The listing builds one solid part. Answer for the finished solid, in the listing's coordinates (mm). A direction names the side the tool comes from. Coordinates: 2 decimals unless noted, no trailing zeros. Order: outer loops, then holes, each group sorted by start corner. A loop starts at its lowest first (then second) coordinate and runs counter-clockwise, first axis right, second up. Notation, with made-up numbers: (32.5, -14.75) -> (44.5, -14.75) arc R24 ccw to (44.5, 0.25) -> close; hole circle Ø9 at (13.25, 54.5). An arc over 180 degrees is marked (long way). One line per question, with ' | ' between items.
from build123d import *

# Parameters (mm, degrees)
BODY_DEPTH          = 160
SKETCH2_R           = 5
PIN_HOLE_DEPTH      = 178.270979012
LPATTERN1_COUNT     = 5
LPATTERN1_PITCH     = 30
SKETCH3_W           = 130
SKETCH3_H           = 170
SKETCH3_W_2         = 100
SKETCH3_H_2         = 150
SPINE_DEPTH         = 40
SKETCH10_W          = 300
SKETCH10_H          = 50
SKETCH10_W_2        = 50
SKETCH10_H_2        = 20
BOSS_EXTRUDE5_DEPTH = 20
CUT_EXTRUDE2_REACH  = 553.549
SKETCH11_W          = 52.942098854
SKETCH11_H          = 11.117065858


with BuildPart() as part:
    # Sketch1 → body (new body)
    with BuildSketch(Plane(origin=(0, 0, 0), x_dir=(1, 0, 0), z_dir=(0, 1, 0))):
        Polygon((65, 20), (-65, 20), (-65, 10), (-55, 10), (-55, -10), (-65, -10), (-65, -20), (65, -20), (65, -10), (55, -10), (55, 10), (65, 10), align=None)
    extrude(amount=BODY_DEPTH)

    # Sketch2 → pin hole (cut, through all)
    with BuildSketch(Plane.XY.offset(20)):
        with Locations((0, 10)):
            Circle(SKETCH2_R)
    pin_hole = extrude(amount=-PIN_HOLE_DEPTH, mode=Mode.SUBTRACT)

    # LPattern1: pin hole ×5
    with Locations(*[(0, i * LPATTERN1_PITCH, 0) for i in range(1, LPATTERN1_COUNT)]):
        add(pin_hole, mode=Mode.SUBTRACT)

    # Sketch3 → spine (add)
    with BuildSketch(Plane.XY.offset(20)):
        with Locations((0, 245)):
            Rectangle(SKETCH3_W, SKETCH3_H)
        with Locations((0, 405)):
            Rectangle(SKETCH3_W_2, SKETCH3_H_2)
    extrude(amount=-SPINE_DEPTH)

    # Sweep4: sweep along a path in Sketch8
    with BuildLine(Plane(origin=(0, 480, 0), x_dir=(1, 0, 0), z_dir=(0, 1, 0))) as sweep4_path:
        ThreePointArc((0, -20), (126.004292483, -12.029696267), (250, 11.754163448))
    # Sketch6<6> → Sweep4 (sweep)
    with BuildSketch(Plane(origin=(0, 0, 0), x_dir=(0, 0, -1), z_dir=(1, 0, 0))):
        Polygon((-70, 480), (-55, 480), (-55, 470), (-35, 470), (-35, 480), (-20, 480), (-20, 430), (-35, 430), (-35, 440), (-55, 440), (-55, 430), (-70, 430), align=None)
    sweep(path=sweep4_path.line)

    # Sketch10 → Boss-Extrude5 (add)
    with BuildSketch(Plane.XY.offset(20)):
        with Locations((0, 455)):
            Rectangle(SKETCH10_W, SKETCH10_H)
        with Locations((-105, 455)):
            Rectangle(SKETCH10_W_2, SKETCH10_H_2, mode=Mode.SUBTRACT)
        with Locations((105, 455)):
            Rectangle(SKETCH10_W_2, SKETCH10_H_2, mode=Mode.SUBTRACT)
    extrude(amount=-BOSS_EXTRUDE5_DEPTH)

    # Sketch11 → Cut-Extrude2 (cut, up to next)
    with BuildSketch(Plane(origin=(0, 480, 0), x_dir=(1, 0, 0), z_dir=(0, 1, 0)), mode=Mode.PRIVATE) as cut_extrude2_sk1:
        with Locations((103.759397545, -17.786929586)):
            Rectangle(SKETCH11_W, SKETCH11_H)
    cut_extrude2_tool1 = extrude(cut_extrude2_sk1.sketch, amount=-CUT_EXTRUDE2_REACH, mode=Mode.PRIVATE) & part.part
    add(cut_extrude2_tool1.solids().sort_by_distance((103.759398, 480, 17.78693))[0], mode=Mode.SUBTRACT)


solid = part.part
Item 1: Section A-A, the plane x = -93 is taken. Give the vertices of the cut face in (y, z), plus the area to 3 significant figures.
Computed values:
outline: (430, 0) -> (445, 0) -> (445, 20) -> (430, 20) -> close; (465, 0) -> (480, 0) -> (480, 20) -> (465, 20) -> close | area: 600 mm^2
Item 2: Section B-B, the plane y = 263 is taken. Give the vertices of the cut face in (x, z).
Computed values:
outline: (-65, -20) -> (65, -20) -> (65, 20) -> (-65, 20) -> close
Item 3: Section C-C, the plane x = 235 is taken. Give the vertices of the cut face in (y, z), plus the area to 3 significant figures.
Computed values:
outline: (430, -8) -> (480, -8) -> (480, 7.42) -> (470, 7.42) -> (470, 27.97) -> (480, 27.97) -> (480, 43.36) -> (430, 43.36) -> (430, 27.97) -> (440, 27.97) -> (440, 7.42) -> (430, 7.42) -> close | area: 2,160 mm^2
Item 4: Each of these flat-tipped pins is pushed along its axis until it touches: pin 1 Ø3.5 at (x, z) = (97.5, 4.5) entering from -Y; pin 2 Ø25 at (x, y) = (106.5, 445) entering from -Z; pin 3 Ø3 at (x, z) = (62, 2) entering from -Y. Where does it stop, or does it pass through?
Computed values:
pin 1: stops at y = 430 | pin 2: stops at z = 0 | pin 3: stops at y = 160
Item 5: For faces 4 (the face through (60, 79, 10)), 5 (the face through (77.288, 455, 18)), 6 (the face through (-65, 199, 0)), determine the directions among +Z, -Z, +X, -X, +Y, -Y from which every point of the face is accessible in a straight line to the end or side of a thin tool.
Computed values:
face 4: +X, -Y | face 5: +Y, -Y | face 6: +Z, -Z, -X, -Y
Item 6: Section D-D, the plane x = 168 is taken. Give the vertices of the cut face in (y, z).
Computed values:
outline: (430, 5.79) -> (480, 5.79) -> (480, 21) -> (470, 21) -> (470, 41.27) -> (480, 41.27) -> (480, 56.47) -> (430, 56.47) -> (430, 41.27) -> (440, 41.27) -> (440, 21) -> (430, 21) -> close
Item 7: Determine the mould class of faces 1 (the face through (130.23, 455, 18)), 2 (the face through (-58, 330, 0)), 3 (the face through (130.462, 454.65, 61.864)) for opening direction X: pulls with the +X half, pulls with the -X half, needs draft (parallel to the pull), parting line crosses it, or undercut.
Computed values:
face 1: undercut | face 2: needs draft | face 3: pulls with the +X half
Item 8: Find the intervals of material crossed by L1, parallel to Y at x = 0, z = -5; L2, parallel to X at y = 413, z = -6; L3, parallel to Z at x = 19, y = 114.5, in increasing order.
Computed values:
L1: y = 0 to 5, 15 to 35, 45 to 65, 75 to 95, 105 to 125, 135 to 480 | L2: x = -50 to 50 | L3: z = -20 to 20
